Print and shaded views of the part. All mm, measured from the part's lowest x, y and z. Round coordinates to 2 decimals unless told otherwise and drop trailing zeros. Order: outer loops, then holes, each group sorted by start corner. A loop starts at its lowest first (then second) coordinate and runs counter-clockwise, first axis right, second up. Notation, with made-up numbers: (40, 45) - (68, 45) arc R20 cw to (68, 58) - close; hole circle Ø2 at (51, 22.25). An arc over 180 degrees is marked (long way). Write item = value, one per line.
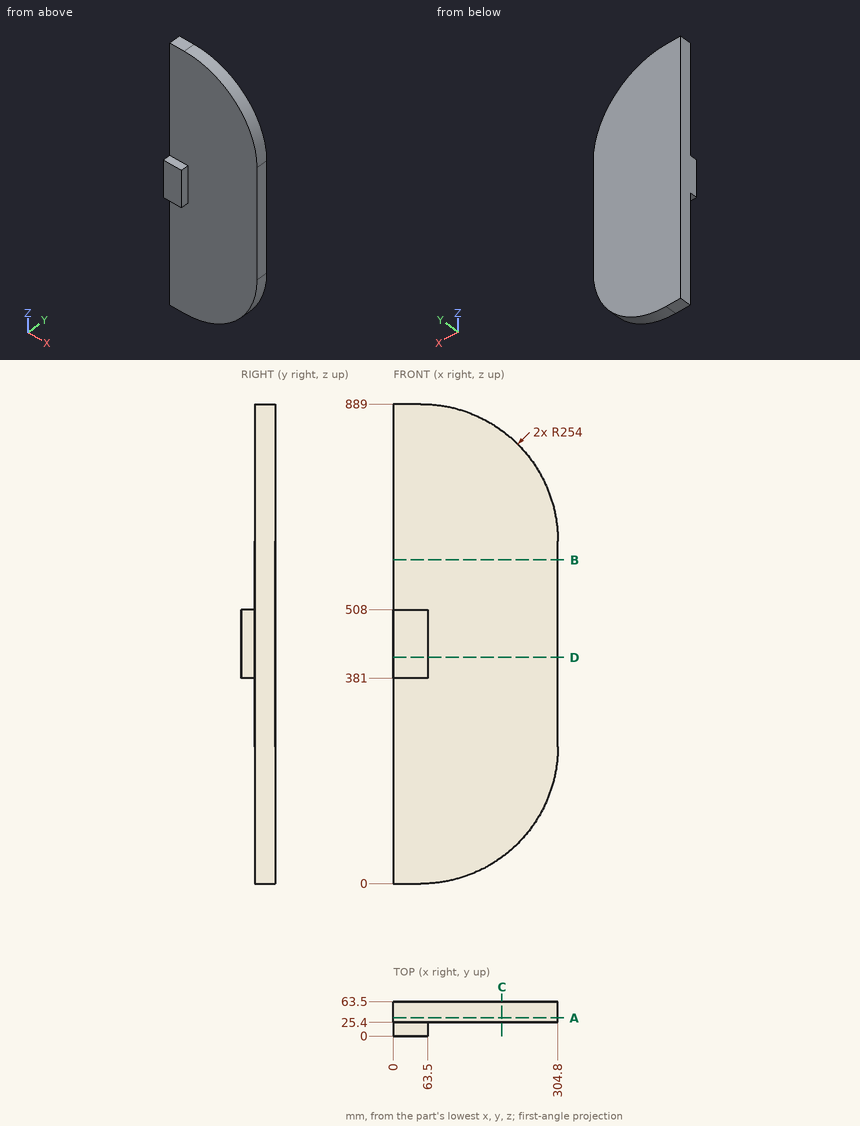
(1) Drop flat-ended pins along their axis: pin 1 (7.5 mm diameter, centred on y = 8.5, z = 416.5, fed in from +X); pin 2 (7.5 mm diameter, centred on x = 26.5, y = 18.5, fed in from -Z); pin 3 (20.5 mm diameter, centred on x = 37, y = 11, fed in from +Z); pin 4 (6 mm diameter, centred on y = 25, z = 306.5, fed in from -X). Give the stop position or say it passes through.
Solved:
pin_1 = 63.5
pin_2 = 381
pin_3 = 508
pin_4 = 0
(2) Band-saw the part on D-D on z = 419.5. List the corners of the cut face in (x, y), plus the area to 3 significant figures.
Solved:
outline = (0, 0) - (63.5, 0) - (63.5, 25.4) - (304.8, 25.4) - (304.8, 63.5) - (0, 63.5) - close
area = 13,200 mm²
(3) Band-saw the part on A-A on y = 33.5. List the corners of the cut face in (x, z).
Solved:
outline = (0, 0) - (50.8, 0) arc R254 ccw to (304.8, 254) - (304.8, 635) arc R254 ccw to (50.8, 889) - (0, 889) - close
(4) Probe line 1 along Y through (x, z) = (23, 659.5); line 2 along X through (y, z) = (12, 466); line 3 along X through (y, z) = (31, 728). List the from-to ranges inside material, lowest first.
Solved:
line_1 = 25.4 to 63.5
line_2 = 0 to 63.5
line_3 = 0 to 287.16
(5) Band-saw the part on B-B on z = 600. List the corners of the cut face in (x, y).
Solved:
outline = (0, 25.4) - (304.8, 25.4) - (304.8, 63.5) - (0, 63.5) - close
(6) Band-saw the part on C-C on x = 201. List the corners of the cut face in (y, z).
Solved:
outline = (25.4, 49.17) - (63.5, 49.17) - (63.5, 839.83) - (25.4, 839.83) - close
